from build123d import *

# Parameters (mm, degrees)
BOSS_EXTRUDE1_DEPTH        = 53.974999999999994
CUT_EXTRUDE1_DEPTH         = 53.974999999999994
CUT_EXTRUDE2_DEPTH         = 40.64
SKETCH4_R                  = 2.0319999999999996
CUT_EXTRUDE3_DEPTH         = 12.699999999999996
CONVERT_SOLID1_DEPTH       = 35.56
CONVERT_SOLID1_START       = 0.640171996
CONVERT_SOLID1_2_OUTLINE_R = 2.032
CONVERT_SOLID1_2_DEPTH     = 0.359828036
CONVERT_SOLID1_START_2     = 52.974999968
CONVERT_SOLID1_3_OUTLINE_W = 15.748000000000001
CONVERT_SOLID1_3_OUTLINE_H = 31.877
CONVERT_SOLID1_3_DEPTH     = 0.241146378
CONVERT_SOLID1_START_3     = 1.000000032
CONVERT_SOLID1_4_OUTLINE_W = 35.56
CONVERT_SOLID1_4_OUTLINE_H = 0.1377071679999986
CONVERT_SOLID1_4_DEPTH     = 51.974999936
CONVERT_SOLID1_5_DEPTH     = 35.56
SCALE1_SCALE               = 1.3


with BuildPart() as part:
    # Sketch1 → Boss-Extrude1 (new body)
    with BuildSketch(Plane(origin=(0, 0, 0), x_dir=(0, 0, -1), z_dir=(1, 0, 0))):
        with BuildLine():
            Line((0, 0), (-44.449999999999996, -5.44e-15))
            Line((-44.449999999999996, -5.44e-15), (-44.449999999999996, 35.55999999999999))
            Line((-44.449999999999996, 35.55999999999999), (0, 35.55999999999999))
            ThreePointArc((0, 35.55999999999999), (17.779999999999994, 17.779999999999994), (0, 0))
        make_face()
    extrude(amount=BOSS_EXTRUDE1_DEPTH)

    # Sketch2 → Cut-Extrude1 (cut)
    with BuildSketch(Plane(origin=(0, 35.55999999999999, 0), x_dir=(1, 0, 0), z_dir=(0, 1, 0))):
        Polygon((0.6401719962352073, 17.998125077829755), (0.6401719962352074, -43.58770713635029), (53.21614634609016, -43.58770713635029), (53.21614634609016, 17.998125077829755), align=None)
    extrude(amount=-CUT_EXTRUDE1_DEPTH, mode=Mode.SUBTRACT)

    # Sketch3 → Cut-Extrude2 (cut)
    with BuildSketch(Plane(origin=(53.974999999999994, 0, 0), x_dir=(0, 0, -1), z_dir=(1, 0, 0))):
        Polygon((-22.098, 25.306389569999986), (9.779, 25.306389569999986), (9.778999999999996, 9.558389569999989), (-22.098, 9.558389569999983), align=None)
    extrude(amount=-CUT_EXTRUDE2_DEPTH, mode=Mode.SUBTRACT)

    # Sketch4 → Cut-Extrude3 (cut)
    with BuildSketch(Plane.ZY):
        with Locations((-1.948939271970541, 17.773350266981094)):
            Circle(SKETCH4_R)
    extrude(amount=-CUT_EXTRUDE3_DEPTH, mode=Mode.SUBTRACT)

    # Convert-Solid1: read off the stored shape, not the designer's step
    # Convert-Solid1 outline → Convert-Solid1 (cut)
    with BuildSketch(Plane(origin=(0, 0, 0), x_dir=(1, 0, 0), z_dir=(0, 1, 0))):
        with BuildLine():
            Line((0, -44.45), (2.000000064, -44.45))
            ThreePointArc((2.000000064, -44.45), (0.585786456, -43.864213544), (0, -42.449999936))
            Line((0, -42.449999936), (0, -44.45))
        make_face()
        with BuildLine():
            Line((53.975, -44.45), (53.975, -42.449999936))
            ThreePointArc((53.975, -42.449999936), (53.389213544, -43.864213544), (51.974999936, -44.45))
            Line((51.974999936, -44.45), (53.975, -44.45))
        make_face()
    extrude(amount=CONVERT_SOLID1_DEPTH, mode=Mode.SUBTRACT)

    # Convert-Solid1 2 outline → Convert-Solid1 2 (add)
    with BuildSketch(Plane.YZ.offset(CONVERT_SOLID1_START)):
        with BuildLine():
            Line((35.56, 43.587707136), (0, 43.587707136))
            Line((0, 43.587707136), (0, 0))
            ThreePointArc((0, 0), (17.78, -17.78), (35.56, 0))
            Line((35.56, 0), (35.56, 43.587707136))
        make_face()
        with Locations((17.773350267, -1.948939272)):
            Circle(CONVERT_SOLID1_2_OUTLINE_R, mode=Mode.SUBTRACT)
    extrude(amount=CONVERT_SOLID1_2_DEPTH)

    # Convert-Solid1 3 outline → Convert-Solid1 3 (add)
    with BuildSketch(Plane.YZ.offset(CONVERT_SOLID1_START_2)):
        with BuildLine():
            Line((35.56, 43.587707136), (0, 43.587707136))
            Line((0, 43.587707136), (0, 0))
            ThreePointArc((0, 0), (17.78, -17.78), (35.56, 0))
            Line((35.56, 0), (35.56, 43.587707136))
        make_face()
        with Locations((17.432389569999998, 6.1594999999999995)):
            Rectangle(CONVERT_SOLID1_3_OUTLINE_W, CONVERT_SOLID1_3_OUTLINE_H, mode=Mode.SUBTRACT)
    extrude(amount=CONVERT_SOLID1_3_DEPTH)

    # Convert-Solid1 4 outline → Convert-Solid1 4 (add)
    with BuildSketch(Plane.YZ.offset(CONVERT_SOLID1_START_3)):
        with Locations((17.78, 43.518853551999996)):
            Rectangle(CONVERT_SOLID1_4_OUTLINE_W, CONVERT_SOLID1_4_OUTLINE_H)
    extrude(amount=CONVERT_SOLID1_4_DEPTH)

    # Convert-Solid1 5 outline → Convert-Solid1 5 (add)
    with BuildSketch(Plane(origin=(0, 0, 0), x_dir=(1, 0, 0), z_dir=(0, 1, 0))):
        with BuildLine():
            Line((1.000000032, -43.449999968), (2.000000064, -43.449999968))
            ThreePointArc((2.000000064, -43.449999968), (1.29289326, -43.15710674), (1.000000032, -42.449999936))
            Line((1.000000032, -42.449999936), (1.000000032, -43.449999968))
        make_face()
        with BuildLine():
            ThreePointArc((52.974999968, -42.449999936), (52.68210674, -43.15710674), (51.974999936, -43.449999968))
            Line((51.974999936, -43.449999968), (52.974999968, -43.449999968))
            Line((52.974999968, -43.449999968), (52.974999968, -42.449999936))
        make_face()
    extrude(amount=CONVERT_SOLID1_5_DEPTH)


with BuildPart() as part_1:
    # Scale1: scaled about (24.607246438, 17.812081852, 25.524433927)
    add(part.part.scale(SCALE1_SCALE).moved(Location((-7.382173931400001, -5.3436245556, -7.657330178100001))))


solid = part_1.part
Model file for the job. Use its own axes, mm. A direction names the side the tool comes from. Round coordinates to 2 decimals unless told otherwise and drop trailing zeros. Order: outer loops, then holes, each group sorted by start corner. A loop starts at its lowest first (then second) coordinate and runs counter-clockwise, first axis right, second up.
(1) Band-saw the part on B-B (z = 19.5). List the corners of the cut face in (x, y), then the cut area to 3 significant figures.
(2) Band-saw the part on D-D (y = 29.5). List the corners of the cut face in (x, z).
(3) Drill centre lines: line 1 (X direction, y = 0.5, z = 12); line 2 (Z direction, x = 21.5, y = 21.5); line 3 (X direction, y = 14.5, z = 16). Where is each one in solid material? Low to high.
(4) Pull direction X, two halves, no side cores. Call faces 1 (the face through (61.485, 28, 18)), 2 (the face through (12, -5.344, 49)), 3 (the face through (-6.082, 17, 9)), 4 (the face through (-7.382, 18, 8)): released by +X, released by -X, zero draft, split by the parting line, or undercut.
(5) Pin check, flat tips, straight feed: pin 1 (1.4 mm diameter, centred on x = 62, y = 14.5, fed in from -Z); pin 2 (4 mm diameter, centred on y = 17.76, z = -10.19, fed in from +X); pin 3 (6 mm diameter, centred on y = 17.76, z = -10.19, fed in from +X); pin 4 (23 mm diameter, centred on y = 17.5, z = 6, fed in from +X). Stop position of each tip, or through.
(6) 3-axis set-ups, long thin cutter, end or side, ignore diameter. For faces 5 (the face through (-6.6, 17.447, 49.386)), 6 (the face through (27, 17, 48.828)): which of +Z, -Z, +X, -X, +Y, -Y reach the whole face in a straight line?
(7) Band-saw the part on A-A (z = 28.5). List the corners of the cut face in (x, y).
(8) Band-saw the part on C-C (y = 11.5). List the corners of the cut face in (x, z).
Verdict:
1. outline: (-7.38, -5.34) - (-6.08, -5.34) - (-6.08, 40.88) - (-7.38, 40.88) - close; (61.49, -5.34) - (62.79, -5.34) - (62.79, 7.08) - (61.49, 7.08) - close; (61.49, 27.55) - (62.79, 27.55) - (62.79, 40.88) - (61.49, 40.88) - close
1. area: 93.6 mm2
2. outline: (-7.38, -27.57) - (-6.08, -27.57) - (-6.08, 47.53) arc R1.3 cw to (-4.78, 48.83) - (60.19, 48.83) arc R1.3 cw to (61.49, 47.53) - (61.49, -27.57) - (62.79, -27.57) - (62.79, 47.53) arc R2.6 ccw to (60.19, 50.13) - (-4.78, 50.13) arc R2.6 ccw to (-7.38, 47.53) - close
3. line 1: x = -7.38 to -6.08, 61.49 to 62.79
3. line 2: z = 48.83 to 50.13
3. line 3: x = -7.38 to -6.08
4. face 1: undercut
4. face 2: zero draft
4. face 3: undercut
4. face 4: released by -X
5. pin 1: stops at z = -30.63
5. pin 2: passes through
5. pin 3: stops at x = -6.08
5. pin 4: stops at x = 62.79
6. face 5: +Z, -X, +Y, -Y
6. face 6: -Z, +Y, -Y
7. outline: (-7.38, -5.34) - (-6.08, -5.34) - (-6.08, 40.88) - (-7.38, 40.88) - close; (61.49, -5.34) - (62.79, -5.34) - (62.79, 40.88) - (61.49, 40.88) - close
8. outline: (-7.38, -29.9) - (-6.08, -29.9) - (-6.08, 47.53) arc R1.3 cw to (-4.78, 48.83) - (60.19, 48.83) arc R1.3 cw to (61.49, 47.53) - (61.49, 21.07) - (62.79, 21.07) - (62.79, 47.53) arc R2.6 ccw to (60.19, 50.13) - (-4.78, 50.13) arc R2.6 ccw to (-7.38, 47.53) - close; (61.49, -29.9) - (62.79, -29.9) - (62.79, -20.37) - (61.49, -20.37) - close
